```python
from build123d import *

# Parameters (mm, degrees)
F2_R = 1.5
F3_R = 1.5
F4_R = 1.5


# Not quite as in the source:
# - a fillet or chamfer that OpenCascade refuses, or shapes differently, is made with other operations: its cross-section is extruded or revolved along the edge and cut away or added


with BuildPart() as f1:
    # F0 (on Front) → F1 (revolve)
    with BuildSketch(Plane.XZ):
        Polygon((21.6, 15.6), (21.6, 0), (24.8, 0), (24.8, 14), (27.3, 16.5), (27.3, 18), (24, 18), align=None)
    revolve(axis=Axis((0, 0, 6.0077635571), (0, 0, -1)))

    # F2
    f2_edges = [f1.edges().sort_by_distance(p)[0] for p in [
        (-21.6, 0, 15.6),
    ]]
    fillet(f2_edges, radius=F2_R)

    # F3
    f3_edges = [f1.edges().sort_by_distance(p)[0] for p in [
        (-24, 0, 18),
    ]]
    fillet(f3_edges, radius=F3_R)

    # F4
    f4_edges = [f1.edges().sort_by_distance(p)[0] for p in [
        (-24.8, 0, 14),
    ]]
    fillet(f4_edges, radius=F4_R)

    # F5: chamfer of 0.1 on 5 edges, made by hand

    # F5_s1 → F5_t2 (revolve, cut)
    with BuildSketch(Plane.XZ):
        Polygon((27.3, 17.9), (27.2, 18), (27.3, 18), align=None)
    revolve(axis=Axis((0, 0, 18), (0, 0, -1)), mode=Mode.SUBTRACT)

    # F5_s3 → F5_t4 (revolve, cut)
    with BuildSketch(Plane.XZ):
        Polygon((27.2707106781, 16.4707106781), (27.3, 16.5414213562), (27.3, 16.5), align=None)
    revolve(axis=Axis((0, 0, 16.5), (0, 0, -1)), mode=Mode.SUBTRACT)

    # F5_s5 → F5_t6 (revolve, cut)
    with BuildSketch(Plane.XZ):
        Polygon((24.8, 0.1), (24.7, 0), (24.8, 0), align=None)
    revolve(axis=Axis((0, 0, 0), (0, 0, -1)), mode=Mode.SUBTRACT)

    # F5_s7 → F5_t8 (revolve, cut)
    with BuildSketch(Plane.XZ):
        Polygon((21.7, 0), (21.6, 0.1), (21.6, 0), align=None)
    revolve(axis=Axis((0, 0, 0), (0, 0, -1)), mode=Mode.SUBTRACT)


solid = f1.part
```
Read the model definition and answer for the solid it produces. Units are mm, in the model's axes. A direction names the side the tool comes from. Round coordinates to 2 decimals unless told otherwise and drop trailing zeros. Loops run counter-clockwise (first coordinate to the right, second up) from the corner with the lowest first, then second, coordinate; pieces in that order, holes last. Notation, with made-up numbers: (12.25, 86.5) -> (43.25, 86.5) arc R34 ccw to (43.25, 123.5) -> close; hole circle Ø8 at (39.5, 23). An arc over 180 degrees is marked (long way). One line per item, written item: value.
1) Flat-ended cylindrical pins translate along their axes: P1, Ø10, axis at x = -13.5, y = -0.5, coming from the +Z side; P2, Ø12, axis at x = 20, y = 17.5, coming from the -Z side; P3, Ø1, axis at x = -19.5, z = 11.5, coming from the +Y side; P4, Ø5, axis at y = -17, z = 16, coming from the -X side. Find the tip coordinate at first contact, or state that the pin passes through.
Answer list:
P1: passes through
P2: stops at z = 0
P3: stops at y = 15.94
P4: stops at x = -23.09
2) The mould has two halves that part along X. Classify faces 1 (the face through (-21.664, 16.612, 17.23)), 2 (the face through (9.97, 19.16, 7.44)), 3 (the face through (-14.2, -20.3, 18)): pulls with the +X half, pulls with the -X half, needs draft (parallel to the pull), parting line crosses it, or undercut.
Answer list:
face 1: parting line crosses it
face 2: undercut
face 3: needs draft
3) For faces 4 (the face through (11.444, 22.002, 6.832)), 5 (the face through (0, 22, 0)), determine the directions among +Z, -Z, +X, -X, +Y, -Y from which every point of the face is accessible in a straight line to the end or side of a thin tool.
Answer list:
face 4: -Z
face 5: -Z, +X, -X, +Y, -Y
4) Consider L1, parallel to X at y = 0, z = 9; L2, parallel to Y at x = 14, z = 4. Determine where each line is inside the solid, lowest interval first. Write a range as [from, to].
Answer list:
L1: x = [-24.8, -21.6], [21.6, 24.8]
L2: y = [-20.47, -16.45], [16.45, 20.47]
5) A cutting plane is placed at A-A (z = 6). Determine the outline of the cut face in (x, y), and give its area (3 significant figures).
Answer list:
outline: circle Ø49.6 at (0, 0); hole circle Ø43.2 at (0, 0)
area: 466 mm²
